Answer from the drawing. Dimensions are ordinates in mm from the lowest x, y and z of the part. A direction names the side the tool comes from. Coordinates: 2 decimals unless noted, no trailing zeros. Loops run counter-clockwise (first coordinate to the right, second up) from the corner with the lowest first, then second, coordinate; pieces in that order, holes last. Notation, with made-up numbers: (4.25, 31) - (27.25, 31) arc R16 cw to (27.25, 45) - close; hole circle Ø6 at (50, 55). An arc over 180 degrees is marked (long way). Write each question's results on one line, items separated by ' | '. Start each with the question number.
1. A cutting plane is placed at C-C on z = 2.5. Determine the outline of the cut face in (x, y).
2. A cutting plane is placed at B-B on x = 25. Determine the outline of the cut face in (y, z).
3. A cutting plane is placed at A-A on z = 5.5. Determine the outline of the cut face in (x, y), then the cut area to 3 significant figures.
4. A cutting plane is placed at D-D on x = 6. Determine the outline of the cut face in (y, z), then the cut area to 4 significant figures.
5. Find the intervals of material crossed by line 1 along Y through (x, z) = (10.25, 5.5); line 2 along X through (y, z) = (19.5, 10); line 3 along Z through (x, y) = (23.9, 20), in increasing order. Write a range as [from, to].
6. Each of these flat-tipped pins is pushed along its axis until it touches: P1, Ø4, axis at x = 30, z = 5.5, coming from the +Y side; P2, Ø3, axis at y = 18.5, z = 3, coming from the +X side; P3, Ø8, axis at x = 18.5, y = 13, coming from the -Z side. Where does it stop, or does it pass through?
7. Determine the mould class of the marked faces 1, 2 and 3 for opening direction Z: released by +Z, released by -Z, zero draft, split by the parting line, or undercut.
8. Which of the six approach directions +Z, -Z, +X, -X, +Y, -Y give full straight-line access (tool end or side, diameter ignored) to the marked faces 4, 5, 6 and 7?
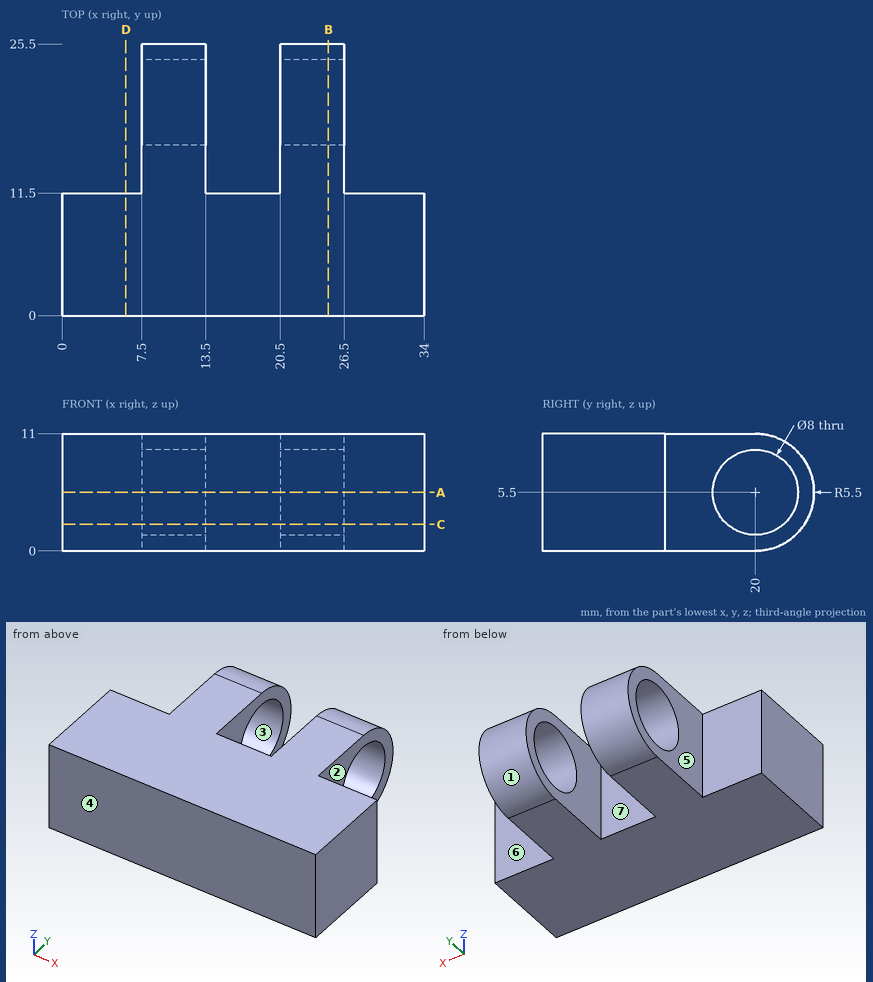
Values:
1) outline: (0, 0) - (34, 0) - (34, 11.5) - (26.5, 11.5) - (26.5, 17.35) - (20.5, 17.35) - (20.5, 11.5) - (13.5, 11.5) - (13.5, 17.35) - (7.5, 17.35) - (7.5, 11.5) - (0, 11.5) - close; (7.5, 22.65) - (13.5, 22.65) - (13.5, 24.61) - (7.5, 24.61) - close; (20.5, 22.65) - (26.5, 22.65) - (26.5, 24.61) - (20.5, 24.61) - close
2) outline: (0, 0) - (20, 0) arc R5.5 ccw to (20, 11) - (0, 11) - close; hole circle Ø8 at (20, 5.5)
3) outline: (0, 0) - (34, 0) - (34, 11.5) - (26.5, 11.5) - (26.5, 16) - (20.5, 16) - (20.5, 11.5) - (13.5, 11.5) - (13.5, 16) - (7.5, 16) - (7.5, 11.5) - (0, 11.5) - close; (7.5, 24) - (13.5, 24) - (13.5, 25.5) - (7.5, 25.5) - close; (20.5, 24) - (26.5, 24) - (26.5, 25.5) - (20.5, 25.5) - close | area: 463 mm^2
4) outline: (0, 0) - (11.5, 0) - (11.5, 11) - (0, 11) - close | area: 126.5 mm^2
5) line 1: [0, 16], [24, 25.5] | line 2: [7.5, 13.5], [20.5, 26.5] | line 3: [0, 1.5], [9.5, 11]
6) P1: y = 11.5 | P2: x = 26.5 | P3: z = 0
7) face 1: split by the parting line | face 2: zero draft | face 3: undercut
8) face 4: +Z, -Z, +X, -X, -Y | face 5: +Z, -Z, -X, +Y | face 6: +Z, -Z, +X, +Y | face 7: +Z, -Z, +Y
